Autodesk Inventor part; units mm, degrees
ref_plane "YZ Plane" through (0, 0, 0) normal (1, 0, 0) x (0, 1, 0)
ref_plane "XZ Plane" through (0, 0, 0) normal (0, 1, 0) x (-1, 0, 0)
ref_plane "XY Plane" through (0, 0, 0) normal (0, 0, 1) x (1, 0, 0)
sketch "Sketch1" plane through (0, 0, 0) normal (0, 0, 1) x (1, 0, 0)
  line L0 (-6.35, -3.6662) -> (-6.35, 3.6662)
  line L1 (-6.35, 3.6662) -> (0, 7.3323)
  line L2 (0, 7.3323) -> (6.35, 3.6662)
  line L3 (6.35, 3.6662) -> (6.35, -3.6662)
  line L4 (6.35, -3.6662) -> (0, -7.3323)
  line L5 (0, -7.3323) -> (-6.35, -3.6662)
  point P0 (0, 0)
  point P1 (0, 0)
  dimension "Size" = 12.7
extrude "Extrusion1" add sketch "Sketch1" along normal mid plane 79.375
sketch "Sketch3" plane through (0, 0, 39.6875) normal (0, 0, 1) x (1, 0, 0)
  line L0 (-6.35, 3.6662) -> (0, 7.3323) construction
  line L1 (0, 7.3323) -> (6.35, 3.6662) construction
  line L2 (6.35, 3.6662) -> (6.35, -3.6662) construction
  line L3 (6.35, -3.6662) -> (0, -7.3323) construction
  line L4 (0, -7.3323) -> (-6.35, -3.6662) construction
  line L5 (-6.35, -3.6662) -> (-6.35, 3.6662) construction
  point P0 (0, 0)
hole "Hole1" at (0, 0, 39.6875) direction (0, 0, -1) diameter 5.1054 end through all
sketch "Sketch4" plane through (0, 0, 39.6875) normal (0, 0, 1) x (1, 0, 0)
  circle A0 centre (0, 0) radius 2.5527 construction
  line L0 (-6.35, 3.6662) -> (0, 7.3323) construction
  line L1 (0, 7.3323) -> (6.35, 3.6662) construction
  line L2 (6.35, 3.6662) -> (6.35, -3.6662) construction
  line L3 (6.35, -3.6662) -> (0, -7.3323) construction
  line L4 (0, -7.3323) -> (-6.35, -3.6662) construction
  line L5 (-6.35, -3.6662) -> (-6.35, 3.6662) construction
  circle A1 centre (0, 0) radius 6.8771
  circle A2 centre (0, 0) radius 8.89
  dimension "thunder" = 13.7541
  dimension "d16" = 17.78
extrude "Extrusion3" cut sketch "Sketch4" against normal through all
equation "\"bearing\" = 25.4"
properties part number "CL3-011" material "Aluminum 6061"
Check sheet for the modelled part. Datum: model origin and axes. Units: mm. Round coordinates to 2 decimals unless told otherwise and drop trailing zeros. Order: outer loops, then holes, each group sorted by start corner. A loop starts at its lowest first (then second) coordinate and runs counter-clockwise, first axis right, second up. Notation, with made-up numbers: (83.25, -31) -> (103.25, -31) arc R24 ccw to (103.25, -16) -> close; hole circle Ø4 at (73, -4.5). An arc over 180 degrees is marked (long way). Use CSV: the item, a comma, the result in double quotes.
(1) Draft check along Y on faces 1 (the face through (-3, 0, -39.688)), 2 (the face through (-0.767, -2.435, -0.556)), 3 (the face through (0.012, 6.877, 0.556)), 4 (the face through (-0.012, -6.877, 0.556)). Enter one of: pulls with the +Y half, pulls with the -Y half, needs draft (parallel to the pull), parting line crosses it, or undercut.
Worked out:
face 1,"needs draft"
face 2,"undercut"
face 3,"pulls with the +Y half"
face 4,"pulls with the -Y half"
(2) Depth check by flat-ended pin: pin 1 (2 mm diameter, centred on x = -3, z = 8, fed in from -Y); pin 2 (2 mm diameter, centred on x = 4, z = 18.5, fed in from +Y); pin 3 (6 mm diameter, centred on x = 0, y = 0, fed in from +Z); pin 4 (2 mm diameter, centred on y = -4, z = 9, fed in from +X). Enter the tip coordinate at first touch or a pass-through.
Worked out:
pin 1,"y = -6.18"
pin 2,"y = 5.6"
pin 3,"z = 39.69"
pin 4,"x = 6.19"
(3) Cross-section at B-B (y = 0). Record the boundary of the cut face in (x, z), and give its area (3 significant figures).
Worked out:
outline,"(-6.35, -39.69) -> (-2.55, -39.69) -> (-2.55, 39.69) -> (-6.35, 39.69) -> close; (2.55, -39.69) -> (6.35, -39.69) -> (6.35, 39.69) -> (2.55, 39.69) -> close"
area,"603 mm²"
(4) Cross-section at A-A (x = 0). Record the boundary of the cut face in (y, z).
Worked out:
outline,"(-6.88, -39.69) -> (-2.55, -39.69) -> (-2.55, 39.69) -> (-6.88, 39.69) -> close; (2.55, -39.69) -> (6.88, -39.69) -> (6.88, 39.69) -> (2.55, 39.69) -> close"
(5) Material ranges on line 1 along X through (y, z) = (0, -17); line 2 along Y through (x, z) = (0, 12); line 3 along Y through (x, z) = (3.25, 4), recorded low to high. Write a range as from..to.
Worked out:
line 1,"-6.35..-2.55, 2.55..6.35"
line 2,"-6.88..-2.55, 2.55..6.88"
line 3,"-5.46..5.46"
(6) Cross-section at C-C (z = -34.5). Record the boundary of the cut face in (x, y).
Worked out:
outline,"(-6.35, -2.64) arc R6.88 ccw to (-5.46, -4.18) -> (-0.89, -6.82) arc R6.88 ccw to (0.89, -6.82) -> (5.46, -4.18) arc R6.88 ccw to (6.35, -2.64) -> (6.35, 2.64) arc R6.88 ccw to (5.46, 4.18) -> (0.89, 6.82) arc R6.88 ccw to (-0.89, 6.82) -> (-5.46, 4.18) arc R6.88 ccw to (-6.35, 2.64) -> close; hole circle Ø5.11 at (0, 0)"
